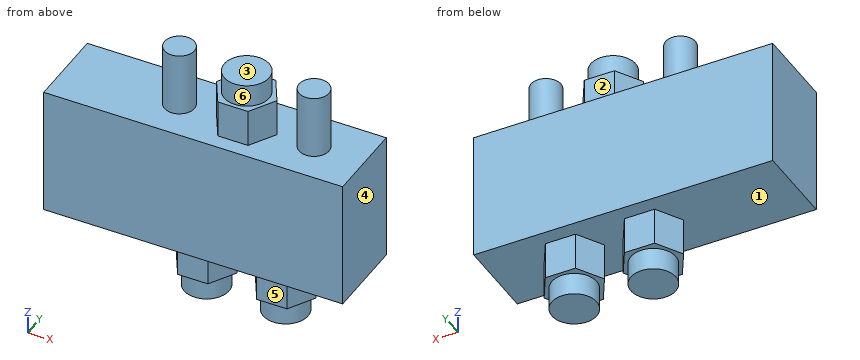
from build123d import *

# Parameters (mm, degrees)
SKETCH1_W           = 80
SKETCH1_H           = 34.5
BOSS_EXTRUDE1_DEPTH = 22
SKETCH2_R           = 4
BOSS_EXTRUDE2_DEPTH = 17
BOSS_EXTRUDE3_DEPTH = 10
BOSS_EXTRUDE6_DEPTH = 10
SKETCH7_R           = 6
BOSS_EXTRUDE7_DEPTH = 6
SKETCH8_R           = 6
BOSS_EXTRUDE8_DEPTH = 6


with BuildPart() as part:
    # Sketch1 → Boss-Extrude1 (new body)
    with BuildSketch(Plane(origin=(0, 0, 0), x_dir=(1, 0, 0), z_dir=(0, 1, 0))):
        with Locations((40, 17.25)):
            Rectangle(SKETCH1_W, SKETCH1_H)
    extrude(amount=BOSS_EXTRUDE1_DEPTH)

    # Sketch2 → Boss-Extrude2 (add)
    with BuildSketch(Plane.XY):
        with Locations((30.5, 11)):
            Circle(SKETCH2_R)
        with Locations((66.5, 11)):
            Circle(SKETCH2_R)
    extrude(amount=BOSS_EXTRUDE2_DEPTH)

    # Sketch3 → Boss-Extrude3 (add)
    with BuildSketch(Plane(origin=(0, 0, -34.5), x_dir=(-1, 0, 0), z_dir=(0, 0, -1))):
        Polygon((-50.834192463, 11), (-54.875644347, 18), (-62.958548116, 18), (-67, 11), (-62.958548116, 4), (-54.875644347, 4), align=None)
        Polygon((-29.668384925, 11), (-33.70983681, 18), (-41.792740578, 18), (-45.834192463, 11), (-41.792740578, 4), (-33.70983681, 4), align=None)
    extrude(amount=BOSS_EXTRUDE3_DEPTH)

    # Sketch6 → Boss-Extrude6 (add)
    with BuildSketch(Plane.XY):
        Polygon((56.582903769, 11), (52.541451884, 18), (44.458548116, 18), (40.417096231, 11), (44.458548116, 4), (52.541451884, 4), align=None)
    extrude(amount=BOSS_EXTRUDE6_DEPTH)

    # Sketch7 → Boss-Extrude7 (add)
    with BuildSketch(Plane.XY.offset(10)):
        with Locations((48.5, 11)):
            Circle(SKETCH7_R)
    extrude(amount=BOSS_EXTRUDE7_DEPTH)

    # Sketch8 → Boss-Extrude8 (add)
    with BuildSketch(Plane(origin=(0, 0, -44.5), x_dir=(-1, 0, 0), z_dir=(0, 0, -1))):
        with Locations((-58.917096231, 11)):
            Circle(SKETCH8_R)
        with Locations((-37.751288694, 11)):
            Circle(SKETCH8_R)
    extrude(amount=BOSS_EXTRUDE8_DEPTH)


solid = part.part
Source: CAD feature listing. Evaluate the final solid. Frame: model axes, mm. Face numbers are marked on the shaded views. A direction names the side the tool comes from. Round coordinates to 2 decimals unless told otherwise and drop trailing zeros. Order: outer loops, then holes, each group sorted by start corner. A loop starts at its lowest first (then second) coordinate and runs counter-clockwise, first axis right, second up. Notation, with made-up numbers: (-32, 50) - (-15, 50) arc R25 cw to (-15, 74) - close; hole circle Ø8 at (-2, 54.5). An arc over 180 degrees is marked (long way). Use a Markdown table: item, result. Add a question column.
1. Set-up query: the marked faces 1, 2 and 3. Return all of +Z, -Z, +X, -X, +Y, -Y with unobstructed straight access to the full face (end or side cutting, diameter ignored); none if empty.
2. Section query B-B (x = 69.5). Return the cut outline in (y, z).
3. Mould query, pull axis X, two halves, no side actions, for the marked faces 4, 5 and 6. Classes: +X half, -X half, draft (parallel to the pull), parting line (faces both ways), or undercut.
4. Section query C-C (y = 19). Return the cut outline in (x, z).
5. Line query: probe 1 along X at (y, z) = (11, -42); probe 2 along Z at (x, y) = (74, 15.5); probe 3 along Z at (x, y) = (31.5, 11.25). Output: solid intervals per line, ascending.
6. Section query A-A (z = -46). Return the cut outline in (x, y).
7. First-contact query: pin 1 (2.5 mm diameter, centred on x = 60.5, z = -39.5, fed in from +Y); pin 2 (3 mm diameter, centred on x = 18.5, y = 6, fed in from -Z); pin 3 (6.5 mm diameter, centred on x = 57, z = -42, fed in from -Y). Flat tips, straight axial feed; report the tip coordinate or a pass-through.
8. Section query D-D (x = 28.5). Return the cut outline in (y, z), then the cut area to 3 significant figures.
Derived:
| question | item | result |
|---|---|---|
| 1 | face 1 | -Z |
| 1 | face 2 | +Z, +X, -X, +Y |
| 1 | face 3 | +Z, +Y, -Y |
| 2 | outline | (0, -34.5) - (22, -34.5) - (22, 0) - (13.65, 0) - (13.65, 17) - (8.35, 17) - (8.35, 0) - (0, 0) - close |
| 3 | face 4 | +X half |
| 3 | face 5 | draft |
| 3 | face 6 | undercut |
| 4 | outline | (0, -34.5) - (80, -34.5) - (80, 0) - (0, 0) - close |
| 5 | probe 1 | 29.67 to 45.83, 50.83 to 67 |
| 5 | probe 2 | -34.5 to 0 |
| 5 | probe 3 | -44.5 to 17 |
| 6 | outline | circle Ø12 at (37.75, 11); circle Ø12 at (58.92, 11) |
| 7 | pin 1 | y = 18 |
| 7 | pin 2 | z = -34.5 |
| 7 | pin 3 | y = 4 |
| 8 | outline | (0, -34.5) - (22, -34.5) - (22, 0) - (14.46, 0) - (14.46, 17) - (7.54, 17) - (7.54, 0) - (0, 0) - close |
| 8 | area | 877 mm2 |
